Autodesk Inventor part; units mm, degrees
ref_plane "YZ Plane" through (0, 0, 0) normal (1, 0, 0) x (0, 1, 0)
ref_plane "XZ Plane" through (0, 0, 0) normal (0, 1, 0) x (-1, 0, 0)
ref_plane "XY Plane" through (0, 0, 0) normal (0, 0, 1) x (1, 0, 0)
sketch "Skizze1" plane through (0, 0, 0) normal (1, 0, 0) x (0, 1, 0)
  line L0 (0, 0) -> (-10, 0) construction
  circle A0 centre (0, 0) radius 1.1
  circle A1 centre (-10, 0) radius 1.1
  arc A2 (-10, 2.5) -> (-10, -2.5) centre (-10, 0) ccw
  line L1 (-10, -2.5) -> (2.5, -2.5)
  line L2 (-10, 2.5) -> (0.5, 2.5)
  arc A3 (2.5, 0.5) -> (0.5, 2.5) centre (0.5, 0.5) ccw
  line L3 (2.5, 0.5) -> (2.5, -2.5)
  dimension "d0" = 10
  dimension "d1" = 2.2
  dimension "d2" = 2.2
  dimension "d3" = 2.5
  dimension "d8" = 2
  dimension "d9" = 2.5
extrude "Extrusion1" add sketch "Skizze1" along normal mid plane 4
chamfer "Fase1" distance 0.5 angle 45 10 edges at (2, 1.9142, 1.9142) (2, -4.75, 2.5) (2, -12.5, 0) (2, -3.75, -2.5) (2, 2.5, -1) (-2, 1.9142, 1.9142) (-2, -4.75, 2.5) (-2, -12.5, 0) (-2, -3.75, -2.5) (-2, 2.5, -1)
sketch "Skizze4" plane through (-1.5, -10, 2.5) normal (0, 0, 1) x (1, 0, 0)
  line L0 (1.5, 15.5) -> (1.5, -5.5) construction
  line L1 (0, 0) -> (3, 0) construction
  line L2 (0.75, 0.4) -> (2.25, 0.4)
  line L3 (2.25, 0.4) -> (2.25, 0)
  line L4 (2.25, 0) -> (0.75, 0)
  line L5 (0.75, 0) -> (0.75, 0.4)
  line L6 (0.75, 0.4) -> (2.25, 0) construction
  line L7 (2.25, 0.4) -> (0.75, 0) construction
  point P0 (1.5, 10)
  point P1 (1.5, 0.2)
  point P2 (1.5, 0)
  dimension "d23" = 0.4
  dimension "d24" = 1.5
extrude "Extrusion3" cut sketch "Skizze4" against normal blind 0.2
equation "\"d2\" = d1"
properties part number "Chipanschlag T0.5"
CAD build for the part. Positions are in the model's coordinates, mm. Coordinates: 2 decimals unless noted, no trailing zeros. Loops run counter-clockwise (first coordinate to the right, second up) from the corner with the lowest first, then second, coordinate; pieces in that order, holes last. Notation, with made-up numbers: (-2.5, 32) -> (25.5, 32) arc R22 ccw to (25.5, 47) -> close; hole circle Ø3 at (16, 8). An arc over 180 degrees is marked (long way). One line per item, written item: value.
1. Slice it at D-D on y = -3. Write the cut outline in (x, z).
Answers:
outline: (-2, -2) -> (-1.5, -2.5) -> (1.5, -2.5) -> (2, -2) -> (2, 2) -> (1.5, 2.5) -> (-1.5, 2.5) -> (-2, 2) -> close
2. Pull direction Y, two halves, no side cores. Call faces 1 (the face through (-0.028, -8.984, 0.421)), 2 (the face through (1.86, 1.65, 1.67)), 3 (the face through (-1.86, -12.14, 0.05)), 4 (the face through (0, -5, 2.5)): pulls with the +Y half, pulls with the -Y half, needs draft (parallel to the pull), parting line crosses it, or undercut.
Answers:
face 1: undercut
face 2: pulls with the +Y half
face 3: pulls with the -Y half
face 4: needs draft
3. Slice it at B-B on z = 0. Write the cut outline in (x, y), and give its area (3 significant figures).
Answers:
outline: (-2, -12) -> (-1.5, -12.5) -> (1.5, -12.5) -> (2, -12) -> (2, -11.1) -> (-2, -11.1) -> close; (-2, -8.9) -> (2, -8.9) -> (2, -1.1) -> (-2, -1.1) -> close; (-2, 1.1) -> (2, 1.1) -> (2, 2) -> (1.5, 2.5) -> (-1.5, 2.5) -> (-2, 2) -> close
area: 41.9 mm^2
4. Flat gauge pin, fed straight in: P1, Ø1.8, axis at y = 0, z = 0, coming from the +X side. Where does the tip first touch, or does it go through?
Answers:
P1: passes through
5. Slice it at A-A on y = 0. Write the cut outline in (x, z), and give its area (3 significant figures).
Answers:
outline: (-2, -2) -> (-1.5, -2.5) -> (1.5, -2.5) -> (2, -2) -> (2, -1.1) -> (-2, -1.1) -> close; (-2, 1.1) -> (2, 1.1) -> (2, 2) -> (1.5, 2.5) -> (-1.5, 2.5) -> (-2, 2) -> close
area: 10.7 mm^2
6. Slice it at C-C on x = -0.5. Write the cut outline in (y, z).
Answers:
outline: (-10, -2.5) -> (2.5, -2.5) -> (2.5, 0.5) arc R2 ccw to (0.5, 2.5) -> (-9.6, 2.5) -> (-9.6, 2.3) -> (-10, 2.3) -> (-10, 2.5) arc R2.5 ccw to start; hole circle Ø2.2 at (-10, 0); hole circle Ø2.2 at (0, 0)
7. Drill centre lines: line 1 (Y direction, x = 0.45, z = -0.05); line 2 (Y direction, x = -0.8, z = -1); line 3 (Z direction, x = 0.85, y = 0). Where is each one in solid material? Low to high. Write a range as [from, to].
Answers:
line 1: y = [-12.5, -11.1], [-8.9, -1.1], [1.1, 2.5]
line 2: y = [-12.29, -10.46], [-9.54, -0.46], [0.46, 2.5]
line 3: z = [-2.5, -1.1], [1.1, 2.5]
